```python
from build123d import *
from OCP.BRepFilletAPI import BRepFilletAPI_MakeChamfer

# Parameters (mm, degrees)
SKETCH1_R             = 2.15
BOSS_EXTRUDE1_DEPTH   = 5
BOSS_EXTRUDE1_2_DEPTH = 5
SKETCH2_W             = 15
SKETCH2_H             = 5
BOSS_EXTRUDE2_DEPTH   = 15
SKETCH3_W             = 15
SKETCH3_H             = 58.581168228
BOSS_EXTRUDE3_DEPTH   = 5
SKETCH4_R             = 10
BOSS_EXTRUDE4_DEPTH   = 5
SKETCH5_R             = 1.55
CUT_EXTRUDE1_DEPTH    = 5
CHAMFER2_SIZE         = 5
CHAMFER2_SIZE2        = 5.958767963
CHAMFER3_SIZE         = 1


with BuildPart() as part:
    # Sketch1 → Boss-Extrude1 (new body)
    with BuildSketch(Plane(origin=(0, 0, 0), x_dir=(1, 0, 0), z_dir=(0, 1, 0))):
        with BuildLine():
            Line((-7.5, -24.290584114), (-7.5, -39.290584114))
            ThreePointArc((-7.5, -39.290584114), (0, -40), (7.5, -39.290584114))
            Line((7.5, -39.290584114), (7.5, -24.290584114))
            Line((7.5, -24.290584114), (-7.5, -24.290584114))
        make_face()
        with Locations(Location((0, -35, 0), (0, 0, 270))):
            Circle(SKETCH1_R, mode=Mode.SUBTRACT)
    extrude(amount=BOSS_EXTRUDE1_DEPTH)



with BuildPart() as body_2:
    # Sketch1 → Boss-Extrude1 2 (new body)
    with BuildSketch(Plane(origin=(0, 0, 0), x_dir=(1, 0, 0), z_dir=(0, 1, 0))):
        with BuildLine():
            Line((-7.5, 39.290584114), (-7.5, 24.290584114))
            Line((-7.5, 24.290584114), (7.5, 24.290584114))
            Line((7.5, 24.290584114), (7.5, 39.290584114))
            ThreePointArc((7.5, 39.290584114), (0, 40), (-7.5, 39.290584114))
        make_face()
        with Locations(Location((0, 35, 0), (0, 0, 270))):
            Circle(SKETCH1_R, mode=Mode.SUBTRACT)
    extrude(amount=BOSS_EXTRUDE1_2_DEPTH)


with BuildPart() as part_1:
    add(part.part)

    add(body_2.part)  # Boss-Extrude2 merges body 2
    # Sketch2 → Boss-Extrude2 (add)
    with BuildSketch(Plane(origin=(0, 5, 0), x_dir=(1, 0, 0), z_dir=(0, 1, 0))):
        with Locations((0, -26.790584114)):
            Rectangle(SKETCH2_W, SKETCH2_H)
        with Locations((0, 26.790584114)):
            Rectangle(SKETCH2_W, SKETCH2_H)
    extrude(amount=BOSS_EXTRUDE2_DEPTH)

    # Sketch3 → Boss-Extrude3 (add)
    with BuildSketch(Plane(origin=(0, 20, 0), x_dir=(1, 0, 0), z_dir=(0, 1, 0))):
        Rectangle(SKETCH3_W, SKETCH3_H)
    extrude(amount=BOSS_EXTRUDE3_DEPTH)

    # Sketch4 → Boss-Extrude4 (add)
    with BuildSketch(Plane(origin=(0, 25, 0), x_dir=(1, 0, 0), z_dir=(0, 1, 0))):
        Circle(SKETCH4_R)
    extrude(amount=-BOSS_EXTRUDE4_DEPTH)

    # Sketch5 → Cut-Extrude1 (cut)
    with BuildSketch(Plane(origin=(0, 25, 0), x_dir=(1, 0, 0), z_dir=(0, 1, 0))):
        with Locations(Location((0, 7, 0), (0, 0, 270))):
            Circle(SKETCH5_R)
        with Locations(Location((7, 0, 0), (0, 0, 270))):
            Circle(SKETCH5_R)
        with Locations(Location((0, -7, 0), (0, 0, 270))):
            Circle(SKETCH5_R)
        with Locations(Location((-7, 0, 0), (0, 0, 270))):
            Circle(SKETCH5_R)
    extrude(amount=-CUT_EXTRUDE1_DEPTH, mode=Mode.SUBTRACT)

    # Chamfer2: one chamfer whose edges measure the first distance from different faces: ONE call of the kernel's chamfer builder (chamfer() names one face for all edges)
    chamfer2_edges_1 = [part_1.edges().sort_by_distance(p)[0] for p in [
        (0, 20, -24.290584114),
    ]]
    chamfer2_side_1 = [part_1.faces().sort_by_distance(p)[0] for p in [
        (0, 10, -24.290584114),
    ]]
    chamfer2_edges_2 = [part_1.edges().sort_by_distance(p)[0] for p in [
        (0, 20, 24.290584114),
    ]]
    chamfer2_side_2 = [part_1.faces().sort_by_distance(p)[0] for p in [
        (0, 10, 24.290584114),
    ]]
    chamfer2 = BRepFilletAPI_MakeChamfer(part_1.part.solid().wrapped)
    for e in chamfer2_edges_1:
        chamfer2.Add(CHAMFER2_SIZE, CHAMFER2_SIZE2, e.wrapped, chamfer2_side_1[0].wrapped)  # the first distance lies on this face
    for e in chamfer2_edges_2:
        chamfer2.Add(CHAMFER2_SIZE, CHAMFER2_SIZE2, e.wrapped, chamfer2_side_2[0].wrapped)  # the first distance lies on this face
    add(Compound.cast(chamfer2.Shape()), mode=Mode.REPLACE)

    # Chamfer3
    chamfer3_edges = [part_1.edges().sort_by_distance(p)[0] for p in [
        (0, 5, -29.290584114),
        (0, 5, 29.290584114),
    ]]
    chamfer(chamfer3_edges, length=CHAMFER3_SIZE)


solid = part_1.part
```
Input: part model. Units: mm. Frame: model coordinates. A direction names the side the tool comes from. Coordinates: 2 decimals unless noted, no trailing zeros. Write each loop counter-clockwise with the first axis right and the second up, starting at its lowest first coordinate (ties: lowest second). Pieces come first, ordered by that corner, then holes. Notation, with made-up numbers: (-16.5, 0) - (-7.5, 0) arc R32 cw to (-7.5, 38) - close; hole circle Ø9 at (6, 0). An arc over 180 degrees is marked (long way). Put each result on its own line as item: value. Start each with the question number.
1) Cut plane B-B (x = 0). State how many separate pieces and enclosed holes the cut face has, plus the area to 3 significant figures.
2) Cut plane C-C (y = 11). Return the cut outline in (x, z), plus the area to 3 significant figures.
3) Cut plane A-A (z = 35). Return the cut outline in (x, y), plus the area to 3 significant figures.
4) Reachability of faces 1 (the face through (0, 15, 29.291)), 2 (the face through (0, 15, -29.291)), 3 (the face through (-7.5, 15, 25)), 4 (the face through (7.5, 14, -25)), 5 (the face through (-0.105, 17.535, -21.269)) from +Z, -Z, +X, -X, +Y, -Y: full face, straight path, thin tool, end or side. Return the list, or none.
5) Ray query, L1, parallel to X at y = 21.15, z = 0; L2, parallel to X at y = 21.45, z = 7; L3, parallel to Z at x = 1.5, y = 14.25. Return the intervals inside material, ascending.
6) Mould query, pull axis X, two halves, no side actions, for faces 6 (the face through (-7.5, 14, -25)), 7 (the face through (0.65, 2.46, 37.05)), 8 (the face through (0.65, 2.46, -32.95)), 9 (the face through (0, 7, 24.291)). Classes: pulls with the +X half, pulls with the -X half, needs draft (parallel to the pull), parting line crosses it, or undercut.
7) Cut plane D-D (x = -4.75). Return the cut outline in (y, z), plus the area to 3 significant figures.
8) Contact query for flat-ended pins moving along their axis: pin 1 (12.5 mm diameter, centred on y = 9, z = 16, fed in from -X); pin 2 (2 mm diameter, centred on y = 22, z = -26, fed in from +X); pin 3 (1.5 mm diameter, centred on x = 6.5, z = 9.5, fed in from -Y); pin 4 (3 mm diameter, centred on x = -2.5, y = 14.5, fed in from +Z). Output: stop coordinate, or through.
Resolved:
1. separate pieces: 5
1. enclosed holes: 0
1. area: 557 mm2
2. outline: (-7.5, -29.29) - (7.5, -29.29) - (7.5, -24.29) - (-7.5, -24.29) - close; (-7.5, 24.29) - (7.5, 24.29) - (7.5, 29.29) - (-7.5, 29.29) - close
2. area: 150 mm2
3. outline: (-7.5, 0) - (-2.15, 0) - (-2.15, 5) - (-7.5, 5) - close; (2.15, 0) - (7.5, 0) - (7.5, 5) - (2.15, 5) - close
3. area: 53.5 mm2
4. face 1: +Z, +X, -X, +Y
4. face 2: -Z, +X, -X, +Y
4. face 3: +Z, -X, +Y, -Y
4. face 4: -Z, +X, +Y, -Y
4. face 5: +X, -X, -Y
5. L1: x = -10 to -8.55, -5.45 to 5.45, 8.55 to 10
5. L2: x = -7.5 to -1.55, 1.55 to 7.5
5. L3: z = -29.29 to -24.29, 24.29 to 29.29
6. face 6: pulls with the -X half
6. face 7: undercut
6. face 8: undercut
6. face 9: needs draft
7. outline: (0, -39.72) - (5, -39.72) - (5, -30.29) - (6, -29.29) - (25, -29.29) - (25, 29.29) - (6, 29.29) - (5, 30.29) - (5, 39.72) - (0, 39.72) - (0, 24.29) - (15, 24.29) - (20, 18.33) - (20, -18.33) - (15, -24.29) - (0, -24.29) - close
7. area: 628 mm2
8. pin 1: passes through
8. pin 2: stops at x = 7.5
8. pin 3: stops at y = 20
8. pin 4: stops at z = 29.29
